from build123d import *

# Parameters (mm, degrees)
SKETCH3_R          = 1.375
CUT_EXTRUDE1_DEPTH = 2


with BuildPart() as part:
    # Sketch2 → Revolve1 (revolve)
    with BuildSketch(Plane.XY, mode=Mode.PRIVATE) as revolve1_sk:
        Polygon((1.5, 0), (11.624355653, 0), (13.5, 7), (13.5, 11.7), (10.5, 14.7), (4, 14.7), (4, 16.2), (1.5, 16.2), (1.5, 27.7), (0, 27.7), (0, -2.1), (1.5, -2.1), align=None)
    revolve(revolve1_sk.sketch.rotate(Axis((0, -2.1, 0), (0, -1, 0)), 180), axis=Axis((0, -2.1, 0), (0, -1, 0)))

    # Sketch3 → Cut-Extrude1 (cut)
    with BuildSketch(Plane.XZ):
        with Locations((0, 9.5)):
            Circle(SKETCH3_R)
        with Locations((0, -9.5)):
            Circle(SKETCH3_R)
        with Locations((-8, 0)):
            Circle(SKETCH3_R)
        with Locations((8, 0)):
            Circle(SKETCH3_R)
    extrude(amount=-CUT_EXTRUDE1_DEPTH, mode=Mode.SUBTRACT)


solid = part.part
Source: CAD feature listing. Evaluate the final solid. Frame: model axes, mm. A direction names the side the tool comes from. Round coordinates to 2 decimals unless told otherwise and drop trailing zeros. Write each loop counter-clockwise with the first axis right and the second up, starting at its lowest first coordinate (ties: lowest second). Pieces come first, ordered by that corner, then holes. Notation, with made-up numbers: M 74.5,-14.5 L 97.5,-14.5 A14 ccw 97.5,5.5 Z; hole C 48.25,24.25 d4. An arc over 180 degrees is marked long. One line per item, written item: value. Start each with the question number.
Item 1: Section query D-D (y = 10.5). Return the cut outline in (x, z), plus the area to 3 significant figures.
Item 2: Section query C-C (y = 15.5). Return the cut outline in (x, z), plus the area to 3 significant figures.
Item 3: Ray query, L1, parallel to Y at x = -5, z = -0.5; L2, parallel to Y at x = 2.5, z = -2; L3, parallel to Z at x = -8, y = 0.65 (3 decimals). Return the intervals inside material, ascending. Write a range as from..to.
Item 4: Section query A-A (z = 0). Return the cut outline in (x, y) (3 decimals).
Item 5: Pin query (flat end, axial travel): pin 1 (5 mm diameter, centred on x = 9.5, z = -8.5, fed in from -Y); pin 2 (6 mm diameter, centred on y = 16, z = 1, fed in from -X); pin 3 (8 mm diameter, centred on x = -9.5, z = 11, fed in from +Y). Return the tip coordinate at first contact, or that it passes through.
Item 6: Section query B-B (x = 0). Return the cut outline in (y, z) (3 decimals).
Item 7: Set-up query: faces 1 (the flat face through (0, -2.1, 0)), 2 (the cylindrical face through (-9.374, 0.986, 0.06)), 3 (the cylindrical face through (0.867, 15.461, 3.905)). Return all of +Z, -Z, +X, -X, +Y, -Y with unobstructed straight access to the full face (end or side cutting, diameter ignored); none if empty.
Item 8: Mould query, pull axis Z, two halves, no side actions, for faces 4 (the cylindrical face through (2.93, 9.38, 13.18)), 5 (the flat face through (-8, 2, 0)), 6 (the flat face through (0, 27.7, 0)). Classes: pulls with the +Z half, pulls with the -Z half, needs draft (parallel to the pull), parting line crosses it, or undercut.
Result set:
1. outline: C 0,0 d27
1. area: 573 mm²
2. outline: C 0,0 d8
2. area: 50.3 mm²
3. L1: y = 0..14.7
3. L2: y = 0..16.2
3. L3: z = -8.672..-1.375, 1.375..8.672
4. outline: M -13.5,7 L -11.624,0 L -9.375,0 L -9.375,2 L -6.625,2 L -6.625,0 L -1.5,0 L -1.5,-2.1 L 1.5,-2.1 L 1.5,0 L 6.625,0 L 6.625,2 L 9.375,2 L 9.375,0 L 11.624,0 L 13.5,7 L 13.5,11.7 L 10.5,14.7 L 4,14.7 L 4,16.2 L 1.5,16.2 L 1.5,27.7 L -1.5,27.7 L -1.5,16.2 L -4,16.2 L -4,14.7 L -10.5,14.7 L -13.5,11.7 Z
5. pin 1: stops at y = 0
5. pin 2: stops at x = -12.17
5. pin 3: stops at y = 14.67
6. outline: M -2.1,-1.5 L 0,-1.5 L 0,-8.125 L 2,-8.125 L 2,-10.875 L 0,-10.875 L 0,-11.624 L 7,-13.5 L 11.7,-13.5 L 14.7,-10.5 L 14.7,-4 L 16.2,-4 L 16.2,-1.5 L 27.7,-1.5 L 27.7,1.5 L 16.2,1.5 L 16.2,4 L 14.7,4 L 14.7,10.5 L 11.7,13.5 L 7,13.5 L 0,11.624 L 0,10.875 L 2,10.875 L 2,8.125 L 0,8.125 L 0,1.5 L -2.1,1.5 Z
7. face 1: +Z, -Z, +X, -X, -Y
7. face 2: -Y
7. face 3: +Y
8. face 4: parting line crosses it
8. face 5: undercut
8. face 6: needs draft
